Design review of the part built by this model. Coordinates are the model's own, in mm. Face numbers are marked on the shaded views. A direction names the side the tool comes from. Give positions to 0.01 mm unless a question says otherwise; leave off trailing zeros. Loops run counter-clockwise (first coordinate to the right, second up) from the corner with the lowest first, then second, coordinate; pieces in that order, holes last. Notation, with made-up numbers: M 55.25,10.5 L 106.25,10.5 A19 ccw 106.25,40.5 Z; hole C 4.5,-25.5 d6. An arc over 180 degrees is marked long. Use a Markdown table: item, result. Add a question column.
(1) Add section C-C, the plane z = -1.85. Give the boundary of the cut face in (x, y), then the cut area to 3 significant figures.
(2) For probe 1 along X at (y, z) = (0, -0.8); probe 2 along Y at (x, z) = (-27, 0.25); probe 3 along Y at (x, z) = (19.62, -1), list the stretches that pass through material, from the lowest coordinate up.
(3) Add section B-B, the plane y = 3. Give the boundary of the cut face in (x, z), then the cut area to 3 significant figures.
(4) For the marked faces 4, 5 and 6, list the 3-axis set-ups (+Z, -Z, +X, -X, +Y, -Y) from which the entire face can be reached by the end or side of a thin tool; tool diameter is ignored.
(5) Insertion check: pin 1 Ø2 at (y, z) = (2, 1.5) entering from +X; pin 2 Ø4.5 at (x, y) = (13, -1.5) entering from +Z. Each pin has a flat end and moves straight along its axis. Give the tip position at first contact, or say it passes through.
(6) Add section A-A, the plane x = 0. Give the boundary of the cut face in (y, z).
(7) Add section D-D, the plane x = 9. Give the boundary of the cut face in (y, z), then the cut area to 3 significant figures.
(8) Draft analysis for pull direction X (two halves, no side actions). For the marked faces 1, 2 and 3, state which applies: pulls with the +X half, pulls with the -X half, needs draft (parallel to the pull), parting line crosses it, or undercut.
Autodesk Inventor part; units mm, degrees
ref_plane "YZ Plane" through (0, 0, 0) normal (1, 0, 0) x (0, 1, 0)
ref_plane "XZ Plane" through (0, 0, 0) normal (0, 1, 0) x (-1, 0, 0)
ref_plane "XY Plane" through (0, 0, 0) normal (0, 0, 1) x (1, 0, 0)
sketch "Sketch1" plane through (0, 0, 0) normal (0, 0, 1) x (1, 0, 0)
  arc A0 (2.1794, -4.5) -> (2.1794, 4.5) centre (0, 0) ccw
  line L0 (-23, -4.5) -> (-2.1794, -4.5)
  line L1 (23, -4.5) -> (23, 4.5)
  line L2 (23, 4.5) -> (2.1794, 4.5)
  line L3 (-23, 4.5) -> (-23, -4.5)
  line L4 (-23, -4.5) -> (23, 4.5) construction
  line L5 (23, -4.5) -> (-23, 4.5) construction
  line L6 (0, 0) -> (23, 0) construction
  line L7 (0, 0) -> (0, 4.5) construction
  line L8 (23, -8.5) -> (-23, -8.5)
  line L9 (-23, -8.5) -> (-23, 8.5)
  line L10 (-23, 8.5) -> (23, 8.5)
  line L11 (23, 8.5) -> (23, -8.5)
  line L12 (23, -8.5) -> (-23, 8.5) construction
  line L13 (-23, -8.5) -> (23, 8.5) construction
  line L14 (-2.1794, 4.5) -> (-23, 4.5)
  line L15 (2.1794, 4.5) -> (-2.1794, 4.5)
  line L16 (-2.1794, -4.5) -> (2.1794, -4.5)
  line L17 (2.1794, -4.5) -> (23, -4.5)
  arc A1 (-2.1794, -4.5) -> (2.1794, -4.5) centre (0, 0) ccw
  arc A2 (2.1794, 4.5) -> (-2.1794, 4.5) centre (0, 0) ccw
  arc A3 (-2.1794, 4.5) -> (-2.1794, -4.5) centre (0, 0) ccw
  point P0 (7.62, 0)
  point P1 (19.62, 0)
  point P2 (-7.62, 0)
  point P3 (-19.62, 0)
  point P4 (20, 0)
  dimension "d0" = 10
  dimension "d1" = 46
  dimension "d2" = 9
  dimension "d3" = 7.62
  dimension "d4" = 12
  dimension "d5" = 4
extrude "Extrusion1" add sketch "Sketch1" against normal blind 3 contours A0 L2 L1 L17 | L17 L11 L8 L9 L0 A1 | A2 L14 L9 L10 L11 L2 | L0 L3 L14 A3
extrude "Extrusion2" add sketch "Sketch1" along normal blind 2 contours A1 L16 | L17 L11 L8 L9 L0 A1 | A2 L14 L9 L10 L11 L2 | L15 A2
sketch "Sketch2" plane through (0, 0, -3) normal (0, 0, -1) x (-1, 0, 0)
  circle A0 centre (0, 0) radius 5
  line L0 (8, 6) -> (42, 6)
  line L1 (42, 6) -> (42, 1)
  line L2 (42, 1) -> (8, 1)
  line L3 (8, 1) -> (8, 6)
  line L4 (-23, -8.5) -> (23, -8.5)
  line L5 (23, 8.5) -> (-23, 8.5)
  line L6 (-23, 8.5) -> (-23, -8.5)
  line L7 (8, 8.5) -> (8, -8.5)
  line L8 (23, -8.5) -> (23, 8.5)
  line L9 (8, -8.5) -> (23, -8.5)
  line L10 (23, 8.5) -> (23, -8.5)
  line L11 (23, 8.5) -> (8, 8.5)
  dimension "d12" = 8
  dimension "d13" = 34
  dimension "d14" = 5
  dimension "d15" = 1
extrude "Extrusion3" add sketch "Sketch2" against normal up to surface (5 mm away) contours L0 L8 L2 L3 | L0 L1 L2 L8
sketch "Sketch3" plane through (-42, 6, -3) normal (0, 1, 0) x (1, 0, 0)
  line L0 (0, -5) -> (19, -5)
  arc A0 (12.5, -5) -> (3.5, -5) centre (8, -8.9686) ccw
  point P0 (42, -3)
  dimension "d33" = 6
  dimension "d35" = 3.5
  dimension "d36" = 9
extrude "Extrusion4" cut sketch "Sketch3" against normal up to next
pattern_linear "Rectangular Pattern1" count 4 spacing 7 along (0, -1, 0) of "Extrusion3", "Extrusion4" first direction both ways yes
extrude "Extrusion5" add sketch "Sketch2" against normal up to surface (5 mm away) contours L7 L5 L8 L0 | L0 L8 L2 L3 | L2 L8 L4 L7
hole "Hole1" at (7.62, 0, 0) at (19.62, 0, 0) at (-19.62, 0, 0) at (-7.62, 0, 0) direction (0, 0, -1) diameter 1 end through all
fillet "Fillet1" radius 4 3 edges at (-42, -10.5, -3) (-42, 3.5, -3) (-42, -3.5, -3)
properties part number "hand1"
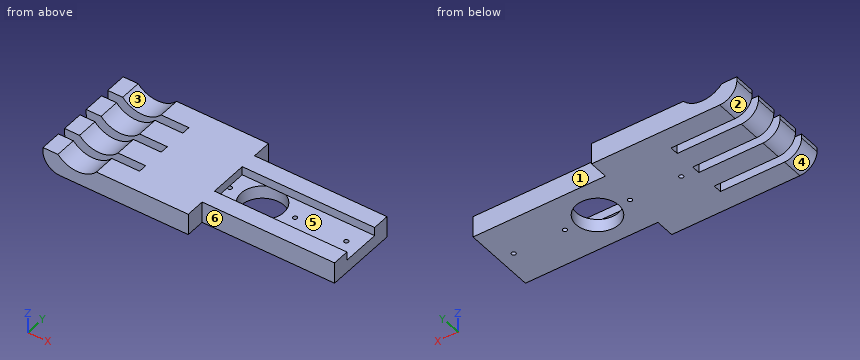
Established:
| question | item | result |
|---|---|---|
| 1 | outline | M -40.81,-13 L -8,-13 L -8,-8.5 L 23,-8.5 L 23,8.5 L -8,8.5 L -8,13 L -40.81,13 L -40.81,8 L -23,8 L -23,6 L -40.81,6 L -40.81,1 L -23,1 L -23,-1 L -40.81,-1 L -40.81,-6 L -23,-6 L -23,-8 L -40.81,-8 Z; hole C -19.62,0 d1; hole C -7.62,0 d1; hole C 0,0 d10; hole C 7.62,0 d1; hole C 19.62,0 d1 |
| 1 | area | 1,190 mm^2 |
| 2 | probe 1 | -23 to -20.12, -19.12 to -8.12, -7.12 to -5, 5 to 7.12, 8.12 to 19.12, 20.12 to 23 |
| 2 | probe 2 | -13 to -8, -6 to -1, 1 to 6, 8 to 13 |
| 2 | probe 3 | -8.5 to -0.5, 0.5 to 8.5 |
| 3 | outline | M -42,1 A4 ccw -38,-3 L -4,-3 L -4,0 L -8,0 L -8,2 L -29.5,2 A6 cw -38.5,2 L -42,2 Z; M 4,-3 L 23,-3 L 23,0 L 4,0 Z |
| 3 | area | 223 mm^2 |
| 4 | face 4 | -Z, -X, +Y, -Y |
| 4 | face 5 | +Z, +X |
| 4 | face 6 | +Z, -Z, +X, -Y |
| 5 | pin 1 | x = -8 |
| 5 | pin 2 | z = 0 |
| 6 | outline | M -8.5,-3 L -5,-3 L -5,0 L -4.5,0 L -4.5,2 L -8.5,2 Z; M 4.5,0 L 5,0 L 5,-3 L 8.5,-3 L 8.5,2 L 4.5,2 Z |
| 7 | outline | M -8.5,-3 L 8.5,-3 L 8.5,2 L 4.5,2 L 4.5,0 L -4.5,0 L -4.5,2 L -8.5,2 Z |
| 7 | area | 67.0 mm^2 |
| 8 | face 1 | needs draft |
| 8 | face 2 | pulls with the -X half |
| 8 | face 3 | undercut |
